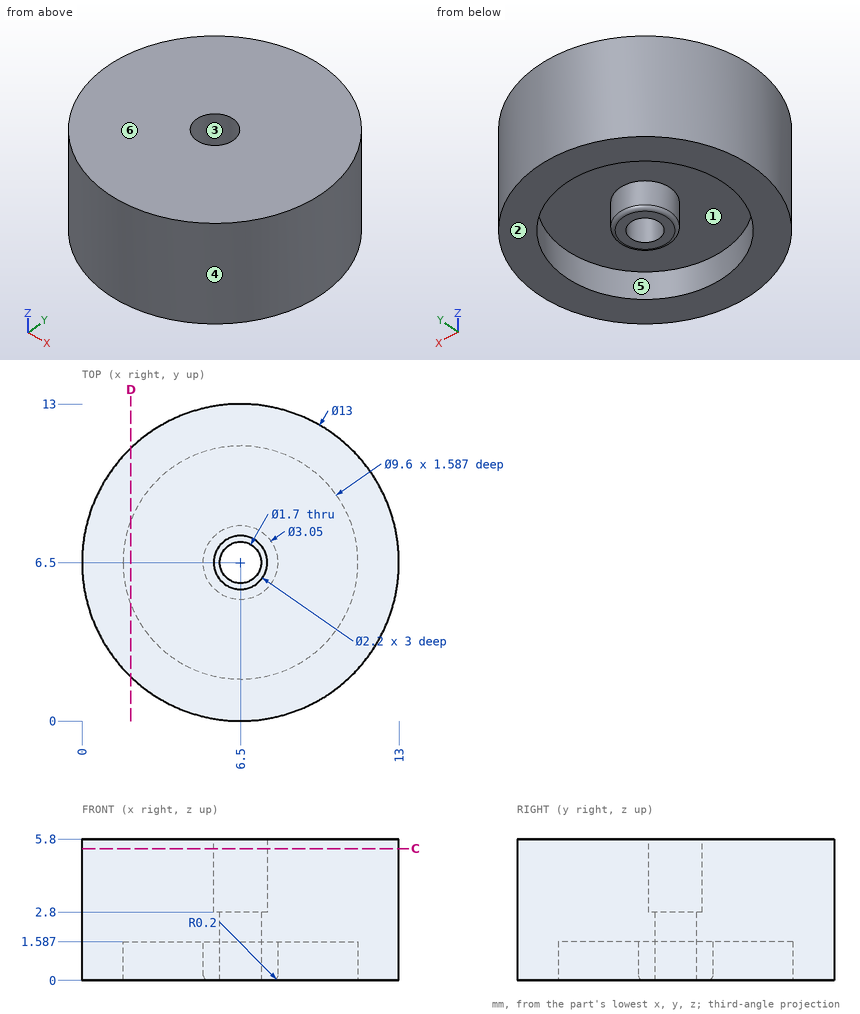
Can you work these out from the drawing? Everything is in mm from the part's minimum corner. A direction names the side the tool comes from. Round coordinates to 2 decimals unless told otherwise and drop trailing zeros. Loops run counter-clockwise (first coordinate to the right, second up) from the corner with the lowest first, then second, coordinate; pieces in that order, holes last. Notation, with made-up numbers: (-6.5, -36) -> (25.5, -36) arc R20 ccw to (25.5, -16) -> close; hole circle Ø10 at (42, 21). An arc over 180 degrees is marked (long way). Answer in a Markdown table with one row per item.
Item 1: Will these pins go through, and if not, where does the flat tip stop? P1, Ø1.8, axis at x = 6.5, y = 6.5, coming from the -Z side; P2, Ø1, axis at y = 4.5, z = 4, coming from the +X side (1 decimal); P3, Ø3, axis at y = 11.5, z = 1, coming from the -X side; P4, Ø1.5, axis at x = 6.5, y = 6.5, coming from the -Z side (1 decimal).
Answer block:
| item | result |
|---|---|
| P1 | z = 0 |
| P2 | x = 12.8 |
| P3 | x = 1.02 |
| P4 | through |
Item 2: On a 3-axis mill with a long thin cutter (end or side, diameter ignored), from which of +Z, -Z, +X, -X, +Y, -Y can I reach the whole of each face in a straight line? I mean the marked faces 1, 2 and 3. Say none if no direction works.
Answer block:
| item | result |
|---|---|
| face 1 | -Z |
| face 2 | -Z, +X, -X, +Y, -Y |
| face 3 | +Z |
Item 3: Suppose I cut it at C-C, the plane z = 5.4. List the corners of the cut face in (x, y) for me.
Answer block:
| item | result |
|---|---|
| outline | circle Ø13 at (6.5, 6.5); hole circle Ø2.2 at (6.5, 6.5) |
Item 4: If I drill on probe 1 along Z at (x, y) = (8, 4.75); probe 2 along Y at (x, z) = (6.5, 3.4); probe 3 along X at (y, z) = (3.5, 0.35) (1 decimal), over which ranges is the centre line in solid material (lowest first)?
Answer block:
| item | result |
|---|---|
| probe 1 | 1.59 to 5.8 |
| probe 2 | 0 to 5.4, 7.6 to 13 |
| probe 3 | 0.7 to 2.8, 10.2 to 12.3 |
Item 5: We'd pull the mould along Y, two halves only. Please class the marked faces 4, 5 and 6: released by +Y, released by -Y, zero draft, split by the parting line, or undercut.
Answer block:
| item | result |
|---|---|
| face 4 | split by the parting line |
| face 5 | undercut |
| face 6 | zero draft |
Item 6: Suppose I cut it at D-D, the plane x = 2. List the corners of the cut face in (y, z) for me.
Answer block:
| item | result |
|---|---|
| outline | (1.81, 0) -> (4.83, 0) -> (4.83, 1.59) -> (8.17, 1.59) -> (8.17, 0) -> (11.19, 0) -> (11.19, 5.8) -> (1.81, 5.8) -> close |
